Source: CAD feature listing. Evaluate the final solid. Frame: model axes, mm. Give positions to 0.01 mm unless a question says otherwise; leave off trailing zeros. Order: outer loops, then holes, each group sorted by start corner. A loop starts at its lowest first (then second) coordinate and runs counter-clockwise, first axis right, second up.
Autodesk Inventor part; units mm, degrees
ref_plane "YZ Plane" through (0, 0, 0) normal (1, 0, 0) x (0, 1, 0)
ref_plane "XZ Plane" through (0, 0, 0) normal (0, 1, 0) x (-1, 0, 0)
ref_plane "XY Plane" through (0, 0, 0) normal (0, 0, 1) x (1, 0, 0)
sketch "Skizze_1" plane through (0, 0, 0) normal (0, 0, 1) x (1, 0, 0)
  line L0 (-17.5, 0) -> (-17.5, -1)
  line L1 (-17.5, -1) -> (-13.5, -1)
  line L2 (-13.5, -1) -> (-13.5, -7.5)
  line L3 (-13.5, -7.5) -> (13.5, -7.5)
  line L4 (13.5, -7.5) -> (13.5, -1)
  line L5 (13.5, -1) -> (17.5, -1)
  line L6 (17.5, -1) -> (17.5, 0)
  line L7 (17.5, 0) -> (12.5, 0)
  line L8 (12.5, 0) -> (12.5, -6.5)
  line L9 (12.5, -6.5) -> (-12.5, -6.5)
  line L10 (-12.5, -6.5) -> (-12.5, 0)
  line L11 (-12.5, 0) -> (-17.5, 0)
extrude "Extrusion1" add sketch "Skizze_1" along normal blind 250
sketch "sketch_roundrect_1" plane through (0, 0, 0) normal (0, 1, 0) x (-1, 0, 0)
  arc A0 (2.6, 9.9) -> (-2.6, 9.9) centre (0, 9.9) ccw
  line L0 (-2.6, 9.9) -> (-2.6, -9.9)
  arc A1 (-2.6, -9.9) -> (2.6, -9.9) centre (0, -9.9) ccw
  line L1 (2.6, -9.9) -> (2.6, 9.9)
extrude "Extrusion2" cut sketch "sketch_roundrect_1" against normal blind 50
sketch "sketch_roundrect_2" plane through (0, 0, 0) normal (0, 1, 0) x (-1, 0, 0)
  arc A0 (2.6, 45.9) -> (-2.6, 45.9) centre (0, 45.9) ccw
  line L0 (-2.6, 45.9) -> (-2.6, 26.1)
  arc A1 (-2.6, 26.1) -> (2.6, 26.1) centre (0, 26.1) ccw
  line L1 (2.6, 26.1) -> (2.6, 45.9)
extrude "Extrusion3" cut sketch "sketch_roundrect_2" against normal blind 50
sketch "sketch_roundrect_3" plane through (0, 0, 0) normal (0, 1, 0) x (-1, 0, 0)
  arc A0 (2.6, 81.9) -> (-2.6, 81.9) centre (0, 81.9) ccw
  line L0 (-2.6, 81.9) -> (-2.6, 62.1)
  arc A1 (-2.6, 62.1) -> (2.6, 62.1) centre (0, 62.1) ccw
  line L1 (2.6, 62.1) -> (2.6, 81.9)
extrude "Extrusion4" cut sketch "sketch_roundrect_3" against normal blind 50
sketch "sketch_roundrect_4" plane through (0, 0, 0) normal (0, 1, 0) x (-1, 0, 0)
  arc A0 (2.6, 117.9) -> (-2.6, 117.9) centre (0, 117.9) ccw
  line L0 (-2.6, 117.9) -> (-2.6, 98.1)
  arc A1 (-2.6, 98.1) -> (2.6, 98.1) centre (0, 98.1) ccw
  line L1 (2.6, 98.1) -> (2.6, 117.9)
extrude "Extrusion5" cut sketch "sketch_roundrect_4" against normal blind 50
sketch "sketch_roundrect_5" plane through (0, 0, 0) normal (0, 1, 0) x (-1, 0, 0)
  arc A0 (2.6, 153.9) -> (-2.6, 153.9) centre (0, 153.9) ccw
  line L0 (-2.6, 153.9) -> (-2.6, 134.1)
  arc A1 (-2.6, 134.1) -> (2.6, 134.1) centre (0, 134.1) ccw
  line L1 (2.6, 134.1) -> (2.6, 153.9)
extrude "Extrusion6" cut sketch "sketch_roundrect_5" against normal blind 50
sketch "sketch_roundrect_6" plane through (0, 0, 0) normal (0, 1, 0) x (-1, 0, 0)
  arc A0 (2.6, 189.9) -> (-2.6, 189.9) centre (0, 189.9) ccw
  line L0 (-2.6, 189.9) -> (-2.6, 170.1)
  arc A1 (-2.6, 170.1) -> (2.6, 170.1) centre (0, 170.1) ccw
  line L1 (2.6, 170.1) -> (2.6, 189.9)
extrude "Extrusion7" cut sketch "sketch_roundrect_6" against normal blind 50
sketch "sketch_roundrect_7" plane through (0, 0, 0) normal (0, 1, 0) x (-1, 0, 0)
  arc A0 (2.6, 225.9) -> (-2.6, 225.9) centre (0, 225.9) ccw
  line L0 (-2.6, 225.9) -> (-2.6, 206.1)
  arc A1 (-2.6, 206.1) -> (2.6, 206.1) centre (0, 206.1) ccw
  line L1 (2.6, 206.1) -> (2.6, 225.9)
extrude "Extrusion8" cut sketch "sketch_roundrect_7" against normal blind 50
sketch "sketch_roundrect_8" plane through (0, 0, 0) normal (0, 1, 0) x (-1, 0, 0)
  arc A0 (2.6, 261.9) -> (-2.6, 261.9) centre (0, 261.9) ccw
  line L0 (-2.6, 261.9) -> (-2.6, 242.1)
  arc A1 (-2.6, 242.1) -> (2.6, 242.1) centre (0, 242.1) ccw
  line L1 (2.6, 242.1) -> (2.6, 261.9)
extrude "Extrusion9" cut sketch "sketch_roundrect_8" against normal blind 50
properties part number "WAGO_210-112250"
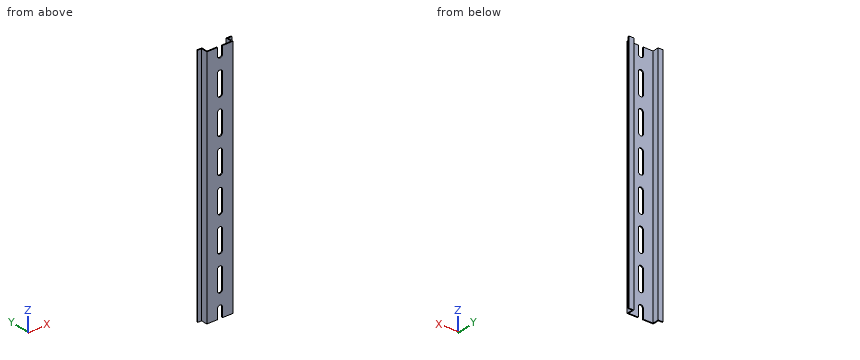
1) Section query C-C, the plane z = 20. Return the cut outline in (x, y), and give its area (3 significant figures).
Report:
outline: (-17.5, -1) - (-13.5, -1) - (-13.5, -7.5) - (13.5, -7.5) - (13.5, -1) - (17.5, -1) - (17.5, 0) - (12.5, 0) - (12.5, -6.5) - (-12.5, -6.5) - (-12.5, 0) - (-17.5, 0) - close
area: 48.0 mm2
2) Section query A-A, the plane y = -5. Return the cut outline in (x, z), and give its area (3 significant figures).
Report:
outline: (-13.5, 0) - (-12.5, 0) - (-12.5, 250) - (-13.5, 250) - close; (12.5, 0) - (13.5, 0) - (13.5, 250) - (12.5, 250) - close
area: 500 mm2
3) Section query B-B, the plane z = 148. Return the cut outline in (x, y).
Report:
outline: (-17.5, -1) - (-13.5, -1) - (-13.5, -7.5) - (-2.6, -7.5) - (-2.6, -6.5) - (-12.5, -6.5) - (-12.5, 0) - (-17.5, 0) - close; (2.6, -7.5) - (13.5, -7.5) - (13.5, -1) - (17.5, -1) - (17.5, 0) - (12.5, 0) - (12.5, -6.5) - (2.6, -6.5) - close
4) Pin query (flat end, axial travel): pin 1 (0.5 mm diameter, centred on y = -7, z = 32.5, fed in from -X); pin 2 (2 mm diameter, centred on y = -2.5, z = 225, fed in from +X); pin 3 (12 mm diameter, centred on x = 4.5, z = 84, fed in from +Y). Return the tip coordinate at first contact, or that it passes through.
Report:
pin 1: stops at x = -13.5
pin 2: stops at x = 13.5
pin 3: stops at y = -6.5
5) Material intervals for L1, parallel to X at y = -5, z = 31.5; L2, parallel to X at y = -0.5, z = 109; L3, parallel to Y at x = 11, z = 147, sorted ascending.
Report:
L1: x = -13.5 to -12.5, 12.5 to 13.5
L2: x = -17.5 to -12.5, 12.5 to 17.5
L3: y = -7.5 to -6.5
